Can you work these out from the model? Positions are in its coordinate system, mm. Round coordinates to 2 decimals unless told otherwise and drop trailing zeros. Loops run counter-clockwise (first coordinate to the right, second up) from the corner with the lowest first, then second, coordinate; pieces in that order, holes last.
```python
from build123d import *

# Parameters (mm, degrees)
SKETCH1_R           = 1.5
SKETCH1_W           = 3
SKETCH1_H           = 10
BOSS_EXTRUDE2_DEPTH = 3


with BuildPart() as part:
    # Sketch1 → Boss-Extrude2 (new body)
    with BuildSketch(Plane(origin=(0, 0, 0), x_dir=(1, 0, 0), z_dir=(0, 1, 0))):
        with BuildLine():
            Line((-42, 30.22741889), (-42, 14.22741889))
            ThreePointArc((-42, 14.22741889), (-41.414213562, 12.813205328), (-40, 12.22741889))
            Line((-40, 12.22741889), (-39, 12.22741889))
            ThreePointArc((-39, 12.22741889), (-36.878679656, 11.348739234), (-36, 9.22741889))
            Line((-36, 9.22741889), (-36, 1.22741889))
            ThreePointArc((-36, 1.22741889), (-36.878679656, -0.893901454), (-39, -1.77258111))
            Line((-39, -1.77258111), (-40, -1.77258111))
            ThreePointArc((-40, -1.77258111), (-41.414213562, -2.358367548), (-42, -3.77258111))
            Line((-42, -3.77258111), (-42, -10.77258111))
            ThreePointArc((-42, -10.77258111), (-40.828427125, -13.601008235), (-38, -14.77258111))
            Line((-38, -14.77258111), (7, -14.77258111))
            ThreePointArc((7, -14.77258111), (8.414213562, -14.186794672), (9, -12.77258111))
            ThreePointArc((9, -12.77258111), (13, -8.77258111), (17, -12.77258111))
            ThreePointArc((17, -12.77258111), (17.585786438, -14.186794672), (19, -14.77258111))
            Line((19, -14.77258111), (38, -14.77258111))
            ThreePointArc((38, -14.77258111), (40.828427125, -13.601008235), (42, -10.77258111))
            Line((42, -10.77258111), (42, 30.22741889))
            ThreePointArc((42, 30.22741889), (40.828427125, 33.055846015), (38, 34.22741889))
            Line((38, 34.22741889), (-38, 34.22741889))
            ThreePointArc((-38, 34.22741889), (-40.828427125, 33.055846015), (-42, 30.22741889))
        make_face()
        with Locations((38, 30.22741889)):
            Circle(SKETCH1_R, mode=Mode.SUBTRACT)
        with Locations((38, -10.77258111)):
            Circle(SKETCH1_R, mode=Mode.SUBTRACT)
        with Locations((-38, -10.77258111)):
            Circle(SKETCH1_R, mode=Mode.SUBTRACT)
        with Locations((-38, 30.22741889)):
            Circle(SKETCH1_R, mode=Mode.SUBTRACT)
        with Locations((27.5, -1.77258111)):
            Rectangle(SKETCH1_W, SKETCH1_H, mode=Mode.SUBTRACT)
        with Locations((27.5, 18.22741889)):
            Rectangle(SKETCH1_W, SKETCH1_H, mode=Mode.SUBTRACT)
        with Locations((-27.5, 18.22741889)):
            Rectangle(SKETCH1_W, SKETCH1_H, mode=Mode.SUBTRACT)
        with Locations((-27.5, -1.77258111)):
            Rectangle(SKETCH1_W, SKETCH1_H, mode=Mode.SUBTRACT)
        with BuildLine():
            Line((-22, -4.416231871), (-22, 14.871069651))
            ThreePointArc((-22, 14.871069651), (9, 5.22741889), (-22, -4.416231871))
        make_face(mode=Mode.SUBTRACT)
    extrude(amount=BOSS_EXTRUDE2_DEPTH)


solid = part.part
```
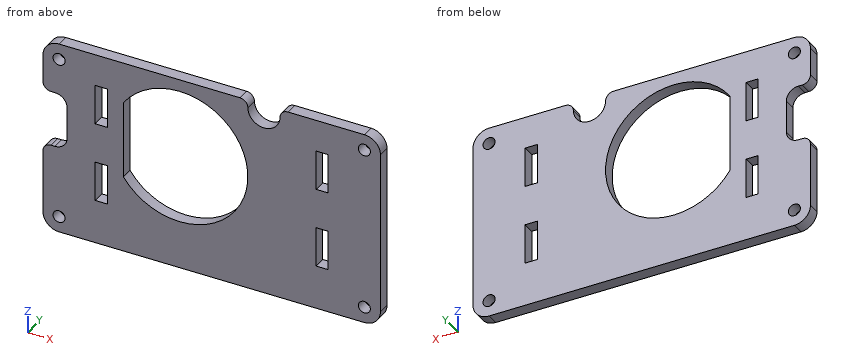
(1) Suppose I cut it at B-B (z = -17). Write out the boundary of the cut face in (x, y).
(2) If I drill on line 1 (Z direction, x = 38, y = 1.15); line 2 (X direction, y = 0.5, z = -30); line 3 (X direction, y = 1.4, z = 5), over which ranges is the centre line in solid material (lowest first)?
(3) Suppose I cut it at A-A (x = -8). Write out the boundary of the cut face in (y, z).
(4) Suppose I cut it at C-C (y = 0.75). Give the number of separate pieces and of enclosed holes in the cut face, then the cut area to 3 significant figures.
(5) For pin 1 (2.5 mm diameter, centred on x = -38, z = -30.23, fed in from -Y); pin 2 (1.1 mm diameter, centred on x = -39.5, y = 2, fed in from -Z), each with a flat end and sliding along its axis, tell me the tip position at first contact or that it passes through.
(6) Suppose I cut it at D-D (x = 13). Write out the boundary of the cut face in (y, z).
Check result:
1. outline: (-42, 0) - (-29, 0) - (-29, 3) - (-42, 3) - close; (-26, 0) - (-20.26, 0) - (-20.26, 3) - (-26, 3) - close; (4.26, 0) - (26, 0) - (26, 3) - (4.26, 3) - close; (29, 0) - (42, 0) - (42, 3) - (29, 3) - close
2. line 1: z = -34.23 to -31.73, -28.73 to 9.27, 12.27 to 14.77
2. line 2: x = -42 to -39.48, -36.52 to 36.52, 39.48 to 42
2. line 3: x = -42 to -29, -26 to -21.58, 5.58 to 26, 29 to 42
3. outline: (0, -34.23) - (3, -34.23) - (3, -22.23) - (0, -22.23) - close; (0, 11.77) - (3, 11.77) - (3, 14.77) - (0, 14.77) - close
4. separate pieces: 1
4. enclosed holes: 9
4. area: 2,960 mm2
5. pin 1: passes through
5. pin 2: stops at z = -34.11
6. outline: (0, -34.23) - (3, -34.23) - (3, 8.77) - (0, 8.77) - close
